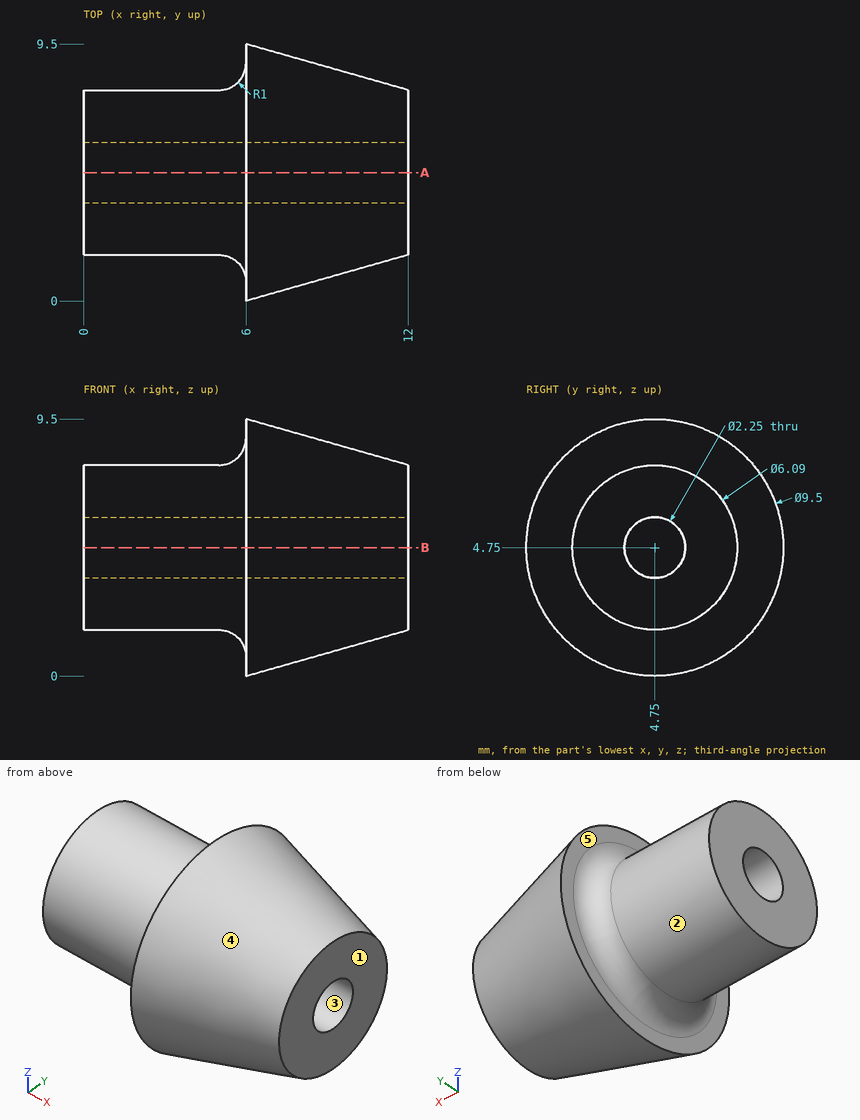
Design review of the part shown in the three views and the two pictorial views. Dimensions are in mm from the part's minimum x, y and z. A direction names the side the tool comes from. Give positions to 0.01 mm unless a question says otherwise; leave off trailing zeros. Loops run counter-clockwise (first coordinate to the right, second up) from the corner with the lowest first, then second, coordinate; pieces in that order, holes last. Notation, with made-up numbers: M 79.25,-3 L 83.25,-3 A22 cw 83.25,28 Z; hole C -2,62.5 d10. An arc over 180 degrees is marked long. Write item = value, one per line.
Q1. Insertion check: pin 1 (2 mm diameter, centred on x = 3.5, z = 8, fed in from +Y); pin 2 (1 mm diameter, centred on x = 2, z = 5.5, fed in from -Y); pin 3 (3 mm diameter, centred on x = 9, z = 4, fed in from -Y). Each pin has a flat end and moves straight along its axis. Give the tip position at first contact, or say it passes through.
Output values:
pin_1 = 6.8
pin_2 = 1.72
pin_3 = 0.46
Q2. We need section A-A (y = 4.75). Give the boundary of the cut face in (x, z) (3 decimals).
Output values:
outline = M 0,1.705 L 5,1.705 A1 cw 6,0.705 L 6,0 L 12,1.705 L 12,3.625 L 0,3.625 Z; M 0,5.875 L 12,5.875 L 12,7.795 L 6,9.5 L 6,8.795 A1 cw 5,7.795 L 0,7.795 Z
Q3. To check wall thickness, follow line 1 (Y direction, x = 1, z = 4.5) (1 decimal); line 2 (Y direction, x = 9.25, z = 4.75) (1 decimal); line 3 (Y direction, x = 7.75, z = 6.5). State the ranges of each line that lie inside material, in increasing order. Write a range as [from, to].
Output values:
line_1 = [1.7, 3.7], [5.8, 7.8]
line_2 = [0.9, 3.6], [5.9, 8.6]
line_3 = [0.87, 8.63]
Q4. For the marked faces 1 and 2, list the 3-axis set-ups (+Z, -Z, +X, -X, +Y, -Y) from which the entire face can be reached by the end or side of a thin tool; tool diameter is ignored.
Output values:
face_1 = +Z, -Z, +X, +Y, -Y
face_2 = -X
Q5. Draft analysis for pull direction Y (two halves, no side actions). For the marked faces 3, 4 and 5, state which applies: +Y half, -Y half, draft (parallel to the pull), parting line (faces both ways), or undercut.
Output values:
face_3 = undercut
face_4 = parting line
face_5 = draft
